Autodesk Fusion 360 part; units mm, degrees
ref_plane "WorkPlane1" through (0, 0, 0) normal (0, 0, 1) x (1, 0, 0)
sketch "Sketch1" plane through (0, 0, 0) normal (0, 0, 1) x (1, 0, 0)
  line L0 (10.25, 10.25) -> (-10.25, 10.25)
  line L1 (-10.25, 10.25) -> (-10.25, -10.25)
  line L2 (-10.25, -10.25) -> (10.25, -10.25)
  line L3 (10.25, -10.25) -> (10.25, 10.25)
  line L4 (10.25, 10.25) -> (-10.25, -10.25) construction
  line L5 (-10.25, 10.25) -> (10.25, -10.25) construction
  line L6 (3.75, 3.75) -> (-3.75, 3.75)
  line L7 (-3.75, 3.75) -> (-3.75, -3.75)
  line L8 (-3.75, -3.75) -> (3.75, -3.75)
  line L9 (3.75, -3.75) -> (3.75, 3.75)
  line L10 (3.75, 3.75) -> (-3.75, -3.75) construction
  line L11 (-3.75, 3.75) -> (3.75, -3.75) construction
  line L12 (8.1, 8.1) -> (-8.1, 8.1)
  line L13 (-8.1, 8.1) -> (-8.1, -8.1)
  line L14 (-8.1, -8.1) -> (8.1, -8.1)
  line L15 (8.1, -8.1) -> (8.1, 8.1)
  line L16 (8.1, 8.1) -> (-8.1, -8.1) construction
  line L17 (-8.1, 8.1) -> (8.1, -8.1) construction
  line L18 (10.25, 10.25) -> (5.55, 10.25)
  line L19 (5.55, 10.25) -> (5.55, 5.55)
  line L20 (5.55, 5.55) -> (10.25, 5.55)
  line L21 (10.25, 5.55) -> (10.25, 10.25)
  line L22 (2.7601, 3.75) -> (5.55, 6.5399)
  line L23 (3.75, 2.7601) -> (6.5399, 5.55)
  line L24 (4.155, 5.145) -> (5.145, 4.155)
  line L25 (-5.55, 5.55) -> (-5.55, 10.25)
  line L26 (-10.25, 5.55) -> (-5.55, 5.55)
  line L27 (-3.75, 2.7601) -> (-6.5399, 5.55)
  line L28 (-2.7601, 3.75) -> (-5.55, 6.5399)
  line L29 (-5.55, -5.55) -> (-10.25, -5.55)
  line L30 (-5.55, -10.25) -> (-5.55, -5.55)
  line L31 (-2.7601, -3.75) -> (-5.55, -6.5399)
  line L32 (-3.75, -2.7601) -> (-6.5399, -5.55)
  line L33 (5.55, -5.55) -> (5.55, -10.25)
  line L34 (10.25, -5.55) -> (5.55, -5.55)
  line L35 (3.75, -2.7601) -> (6.5399, -5.55)
  line L36 (2.7601, -3.75) -> (5.55, -6.5399)
  point P0 (4.65, 4.65)
  dimension "d2" = 20.5
  dimension "d3" = 20.5
  dimension "d4" = 7.5
  dimension "d5" = 7.5
  dimension "d6" = 16.2
  dimension "d7" = 16.2
  dimension "d8" = 4.7
  dimension "d9" = 4.7
  dimension "d10" = 1.4
  dimension "d12" = 360
extrude "Extrude1" add sketch "Sketch1" against normal blind 5 makes body 1
extrude "Extrude2" add sketch "Sketch1" along normal blind 10 draft -1 separate body contours L6 L12 L19 L22 L25 L28 makes body 2
sketch "Sketch2" plane through (0, 0, -5) normal (0, 0, -1) x (1, 0, 0)
  line L0 (10.25, -10.25) -> (10.25, 10.25)
  line L1 (10.25, 10.25) -> (-10.25, 10.25)
  line L2 (-10.25, 10.25) -> (-10.25, -10.25)
  line L3 (-10.25, -10.25) -> (10.25, -10.25)
  circle A0 centre (0, 0) radius 2.1
  line L4 (2.0063, 3.475) -> (-2.0063, 3.475)
  line L5 (-2.0063, 3.475) -> (-4.0126, 0)
  line L6 (-4.0126, 0) -> (-2.0063, -3.475)
  line L7 (-2.0063, -3.475) -> (2.0063, -3.475)
  line L8 (2.0063, -3.475) -> (4.0126, 0)
  line L9 (4.0126, 0) -> (2.0063, 3.475)
  dimension "d17" = 4.2
  dimension "d18" = 3.475
fillet "Fillet1" radius 0.5 6 edges at (2.7239, 3.8373, 5) (-2.7239, 3.8373, 5) (-5.4627, 6.5761, 5) (5.4627, 6.5761, 5) (5.4627, 8.0127, 5) (-5.4627, 8.0127, 5) on bodies 2
pattern_circular "C-Pattern1" count 4 over 360 about axis through (0, 0, 1.75) along (0, 0, 1) of bodies 2 makes body 3 at (-8.0418, 1.6252, 3.3333) makes body 4 at (-1.6252, -8.0418, 3.3333) makes body 5 at (8.0418, -1.6252, 3.3333)
combine "Combine1" operation add target body 5 tool bodies 4 3 2 1
fillet "Fillet2" radius 0.2 4 edges at (10.25, -10.25, -2.5) (10.25, 10.25, -2.5) (-10.25, 10.25, -2.5) (-10.25, -10.25, -2.5) on bodies 5
equation "d18 = ( 6.95 / 2 ) * 1 mm"
The model under review builds one solid part; all positions refer to its coordinate system, in mm. Coordinates: 2 decimals unless noted, no trailing zeros. Write each loop counter-clockwise with the first axis right and the second up, starting at its lowest first coordinate (ties: lowest second). Pieces come first, ordered by that corner, then holes. Notation, with made-up numbers: (32.25, -4) -> (81.25, -4) arc R8 cw to (81.25, 11) -> close; hole circle Ø9 at (39.25, 8). An arc over 180 degrees is marked (long way). Answer in a Markdown table with one row per item.
1. Clearance check with flat-ended pins moving along their axes: pin 1 Ø5 at (x, z) = (5, 3.5) entering from +Y; pin 2 Ø4 at (x, z) = (-3.5, 5.5) entering from +Y; pin 3 Ø2 at (x, z) = (7, 2) entering from +Y. State where each tip first meets the part, or that it passes through.
Answers below:
| item | result |
|---|---|
| pin 1 | stops at y = 8.08 |
| pin 2 | stops at y = 8.04 |
| pin 3 | stops at y = 5.53 |
2. Wall thickness on probe 1 along Y at (x, z) = (-4, 0.75); probe 2 along Z at (x, y) = (0, -0.5); probe 3 along Y at (x, z) = (4.75, 1.25): over which ranges is each line inside the solid? List them lowest first. Write a range as [from, to].
Answers below:
| item | result |
|---|---|
| probe 1 | y = [-8.09, -5.01], [-2.99, 2.99], [5.01, 8.09] |
| probe 2 | z = [-5, 0] |
| probe 3 | y = [-8.08, -5.77], [-3.73, 3.73], [5.77, 8.08] |
3. Draft analysis for pull direction Y (two halves, no side actions). For faces 1 (the flat face through (0, 0, 0)), 2 (the flat face through (0, 10.25, -2)), 3 (the flat face through (-6, 0, 10)), state which applies: +Y half, -Y half, draft (parallel to the pull), parting line (faces both ways), or undercut.
Answers below:
| item | result |
|---|---|
| face 1 | undercut |
| face 2 | +Y half |
| face 3 | draft |
4. We need section C-C, the plane z = 8.5. Give the number of separate pieces and of enclosed holes in the cut face, and give its area (3 significant figures).
Answers below:
| item | result |
|---|---|
| separate pieces | 4 |
| enclosed holes | 0 |
| area | 145 mm^2 |
5. We need section D-D, the plane x = 6. State the section outline as (y, z) points, and give its area (3 significant figures).
Answers below:
| item | result |
|---|---|
| outline | (-10.25, -5) -> (10.25, -5) -> (10.25, 0) -> (5.01, 0) -> (4.76, 10) -> (-4.76, 10) -> (-5.01, 0) -> (-10.25, 0) -> close |
| area | 200 mm^2 |
6. We need section A-A, the plane x = 2. State the section outline as (y, z) points, and give its area (3 significant figures).
Answers below:
| item | result |
|---|---|
| outline | (-10.25, -5) -> (10.25, -5) -> (10.25, 0) -> (8.1, 0) -> (7.93, 10) -> (3.92, 10) -> (3.75, 0) -> (-3.75, 0) -> (-3.92, 10) -> (-7.93, 10) -> (-8.1, 0) -> (-10.25, 0) -> close |
| area | 186 mm^2 |
